from build123d import *

# Parameters (mm, degrees)
BOSS_EXTRUDE1_DEPTH                               = 5.715
SKETCH1_W                                         = 201
SKETCH1_H                                         = 241
CUT_EXTRUDE1_DEPTH                                = 6.715
CSK_FOR_6_FLAT_HEAD_MACHINE_SCREW_100_D           = 3.7973
CSK_FOR_6_FLAT_HEAD_MACHINE_SCREW_100_CSINK_D     = 7.0866
CSK_FOR_6_FLAT_HEAD_MACHINE_SCREW_100_CSINK_ANGLE = 100
CSK_FOR_6_FLAT_HEAD_MACHINE_SCREW_2_D             = 3.7973
CSK_FOR_6_FLAT_HEAD_MACHINE_SCREW_2_CSINK_D       = 7.0866
CSK_FOR_6_FLAT_HEAD_MACHINE_SCREW_2_CSINK_ANGLE   = 100


with BuildPart() as part:
    # Model → Boss-Extrude1 (new body)
    with BuildSketch(Plane.XY):
        Polygon((1148.22, 22.8575), (1152.62, 22.8575), (1152.62, 28.5722), (1164.05, 28.5722), (1164.05, 22.8575), (1175.48, 22.8575), (1175.48, 28.5722), (1186.91, 28.5722), (1186.91, 22.8575), (1198.34, 22.8575), (1198.34, 28.5722), (1209.77, 28.5722), (1209.77, 22.8575), (1221.2, 22.8575), (1221.2, 28.5722), (1232.63, 28.5722), (1232.63, 22.8575), (1244.06, 22.8575), (1244.06, 28.5722), (1255.49, 28.5722), (1255.49, 22.8575), (1266.92, 22.8575), (1266.92, 28.5722), (1278.35, 28.5722), (1278.35, 22.8575), (1289.78, 22.8575), (1289.78, 28.5722), (1301.21, 28.5722), (1301.21, 22.8575), (1312.64, 22.8575), (1312.64, 28.5722), (1324.07, 28.5722), (1324.07, 22.8575), (1335.5, 22.8575), (1335.5, 28.5722), (1346.93, 28.5722), (1346.93, 22.8575), (1358.36, 22.8575), (1358.36, 28.5722), (1369.79, 28.5722), (1369.79, 22.8575), (1374.18, 22.8575), (1379.9, 22.8575), (1379.9, 28.5722), (1379.9, 288.572), (1379.9, 294.287), (1374.18, 294.287), (1369.79, 294.287), (1369.79, 288.572), (1358.36, 288.572), (1358.36, 294.287), (1346.93, 294.287), (1346.93, 288.572), (1335.5, 288.572), (1335.5, 294.287), (1324.07, 294.287), (1324.07, 288.572), (1312.64, 288.572), (1312.64, 294.287), (1301.21, 294.287), (1301.21, 288.572), (1289.78, 288.572), (1289.78, 294.287), (1278.35, 294.287), (1278.35, 288.572), (1266.92, 288.572), (1266.92, 294.287), (1255.49, 294.287), (1255.49, 288.572), (1244.06, 288.572), (1244.06, 294.287), (1232.63, 294.287), (1232.63, 288.572), (1221.2, 288.572), (1221.2, 294.287), (1209.77, 294.287), (1209.77, 288.572), (1198.34, 288.572), (1198.34, 294.287), (1186.91, 294.287), (1186.91, 288.572), (1175.48, 288.572), (1175.48, 294.287), (1164.05, 294.287), (1164.05, 288.572), (1152.62, 288.572), (1152.62, 294.287), (1148.22, 294.287), (1148.22, 288.572), (1148.22, 28.5722), align=None)
    extrude(amount=BOSS_EXTRUDE1_DEPTH)

    # Sketch1 → Cut-Extrude1 (cut, through all)
    with BuildSketch(Plane(origin=(0, 0, 0), x_dir=(-1, 0, 0), z_dir=(0, 0, -1))):
        with Locations((-1264.185, 158.57225)):
            Rectangle(SKETCH1_W, SKETCH1_H)
    extrude(amount=-CUT_EXTRUDE1_DEPTH, mode=Mode.SUBTRACT)

    # CSK for _6 Flat Head Machine Screw _100 (through all)
    with Locations(Plane(origin=(0, 0, 0), x_dir=(-1, 0, 0), z_dir=(0, 0, -1))):
        with Locations((-1301.85166666, 283.822125), (-1226.51833334, 283.822125), (-1226.51833334, 33.322375), (-1301.85166666, 33.322375)):
            CounterSinkHole(CSK_FOR_6_FLAT_HEAD_MACHINE_SCREW_100_D / 2, CSK_FOR_6_FLAT_HEAD_MACHINE_SCREW_100_CSINK_D / 2, counter_sink_angle=CSK_FOR_6_FLAT_HEAD_MACHINE_SCREW_100_CSINK_ANGLE)

    # CSK for _6 Flat Head Machine Screw _ 2 (through all)
    with Locations(Plane(origin=(0, 0, 0), x_dir=(-1, 0, 0), z_dir=(0, 0, -1))):
        with Locations((-1369.435, 246.0721), (-1369.435, 191.0721), (-1369.435, 126.0721), (-1369.435, 71.0721)):
            CounterSinkHole(CSK_FOR_6_FLAT_HEAD_MACHINE_SCREW_2_D / 2, CSK_FOR_6_FLAT_HEAD_MACHINE_SCREW_2_CSINK_D / 2, counter_sink_angle=CSK_FOR_6_FLAT_HEAD_MACHINE_SCREW_2_CSINK_ANGLE)


solid = part.part
Read the model definition and answer for the solid it produces. Units are mm, in the model's axes. A direction names the side the tool comes from. Round coordinates to 2 decimals unless told otherwise and drop trailing zeros. Write each loop counter-clockwise with the first axis right and the second up, starting at its lowest first coordinate (ties: lowest second). Pieces come first, ordered by that corner, then holes.
1. Which of the six approach directions +Z, -Z, +X, -X, +Y, -Y give full straight-line access (tool end or side, diameter ignored) to faces 1 (the face through (1186.91, 291, 3)), 2 (the face through (1364.685, 157, 3)), 3 (the face through (1278.35, 26, 3))?
2. Straight lines are drawn through the part: L1, parallel to Y at x = 1248, z = 2; L2, parallel to X at y = 189, z = 0.4 (3 decimals); L3, parallel to Y at x = 1301, z = 4.1. For each, find the intervals that lie inside material, in ascending order.
3. The part is cut by section C-C, the plane z = 3.5. State how many separate pieces and enclosed holes the cut face has, then the cut area to 3 significant figures.
4. Determine the mould class of faces 4 (the face through (1330, 294.287, 3)), 5 (the face through (1379.9, 157, 3)), 6 (the face through (1232.63, 26, 3)), 7 (the face through (1198.34, 26, 3)) for opening direction X: pulls with the +X half, pulls with the -X half, needs draft (parallel to the pull), parting line crosses it, or undercut.
5. The part is cut by section B-B, the plane y = 56.5. Determine the outline of the cut face in (x, z) (3 decimals), then the cut area to 3 significant figures.
6. The part is cut by section A-A, the plane x = 1274.5. Determine the outline of the cut face in (y, z) (3 decimals), then the cut area to 3 significant figures.
Values:
1. face 1: +Z, -Z, +Y
1. face 2: +Z, -Z
1. face 3: +Z, -Z, -Y
2. L1: y = 28.57 to 38.07, 279.07 to 288.57
2. L2: x = 1148.22 to 1163.685, 1364.685 to 1367.174, 1371.696 to 1379.9
2. L3: y = 28.57 to 31.63, 35.02 to 38.07, 279.07 to 282.13, 285.52 to 288.57
3. separate pieces: 1
3. enclosed holes: 9
3. area: 13,000 mm2
4. face 4: needs draft
4. face 5: pulls with the +X half
4. face 6: undercut
4. face 7: undercut
5. outline: (1148.22, 0) - (1163.685, 0) - (1163.685, 5.715) - (1148.22, 5.715) - close; (1364.685, 0) - (1379.9, 0) - (1379.9, 5.715) - (1364.685, 5.715) - close
5. area: 175 mm2
6. outline: (28.572, 0) - (38.072, 0) - (38.072, 5.715) - (28.572, 5.715) - close; (279.072, 0) - (288.572, 0) - (288.572, 5.715) - (279.072, 5.715) - close
6. area: 109 mm2
